For this review, use the dimensioned drawing (mm, ordinates from the lowest corner) and the shaded views. Coordinates: 2 decimals unless noted, no trailing zeros. Order: outer loops, then holes, each group sorted by start corner. A loop starts at its lowest first (then second) coordinate and runs counter-clockwise, first axis right, second up. Notation, with made-up numbers: (49, 7) -> (86, 7) arc R31 cw to (86, 34) -> close; hole circle Ø4 at (14.25, 42.25). An arc over 180 degrees is marked (long way). Return JSON: item names as keys, results as strings. Group by question number.
Item 1: For line 1 along Y through (x, z) = (44, 28); line 2 along Z through (x, y) = (10, 2.5); line 3 along X through (y, z) = (1.8, 44), list the stretches that pass through material, from the lowest coordinate up.
Item 2: Take a section at A-A (x = 25). Write out the cut boundary in (y, z).
Item 3: Take a section at C-C (z = 25). Write out the cut boundary in (x, y).
Item 4: Take a section at D-D (y = 7.75). Write out the cut boundary in (x, z).
Item 5: Draft analysis for pull direction X (two halves, no side actions). For the marked faces 1, 2 and 3, state which applies: +X half, -X half, draft (parallel to the pull), parting line (faces both ways), or undercut.
Item 6: Insertion check: pin 1 (4 mm diameter, centred on x = 6, z = 25, fed in from -Y); pin 2 (5 mm diameter, centred on x = 25, z = 6, fed in from +Y); pin 3 (1 mm diameter, centred on x = 40.5, y = 2, fed in from -Z); pin 4 (6 mm diameter, centred on x = 31.5, y = 3.5, fed in from -Z). Each pin has a flat end and moves straight along its axis. Give the tip position at first contact, or say it passes through.
Item 7: Take a section at B-B (z = 44). Write out the cut boundary in (x, y), then the cut area to 3 significant figures.
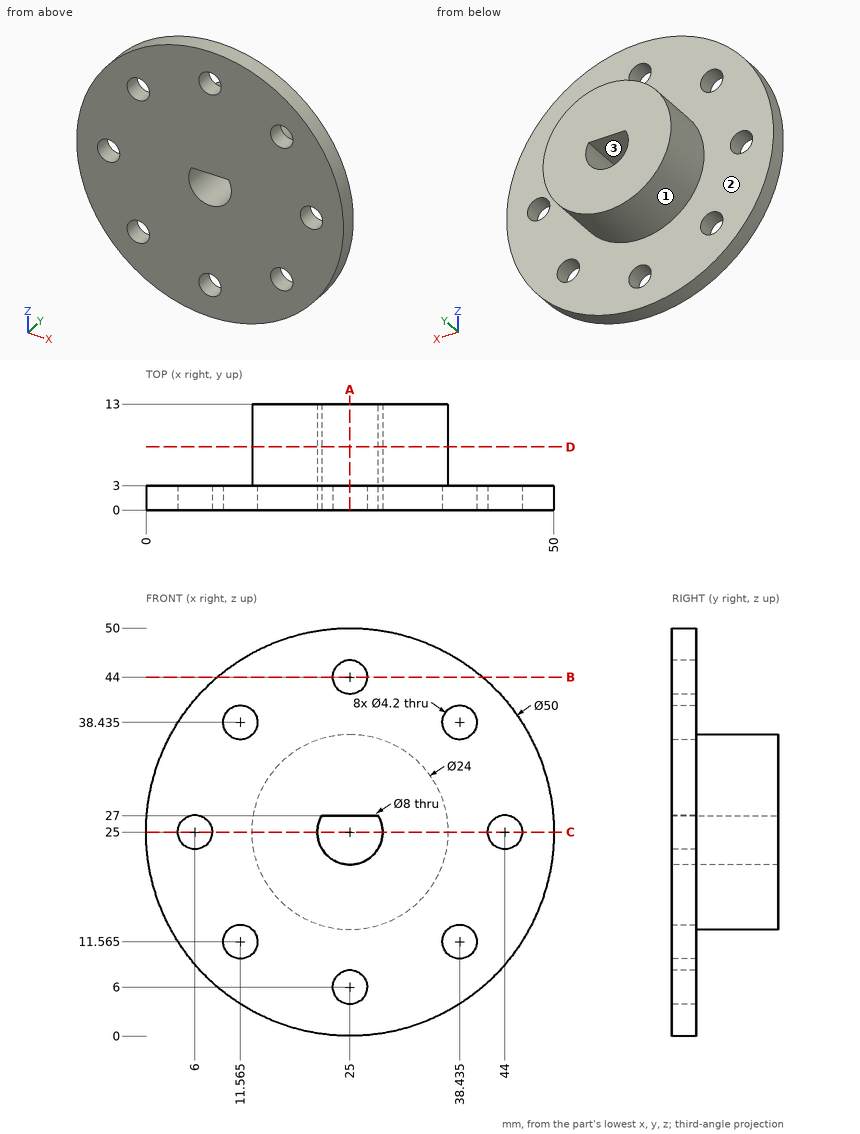
Findings below:
{
 "1": {"line 1": "y = 0 to 3", "line 2": "z = 5 to 10.16, 12.97 to 37.03, 39.84 to 45", "line 3": "x = 8.75 to 22.9, 27.1 to 41.25"},
 "2": {"outline": "(0, 0) -> (3, 0) -> (3, 3.9) -> (0, 3.9) -> close; (0, 8.1) -> (3, 8.1) -> (3, 13) -> (13, 13) -> (13, 21) -> (0, 21) -> close; (0, 27) -> (13, 27) -> (13, 37) -> (3, 37) -> (3, 41.9) -> (0, 41.9) -> close; (0, 46.1) -> (3, 46.1) -> (3, 50) -> (0, 50) -> close"},
 "3": {"outline": "(0, 0) -> (3.9, 0) -> (3.9, 3) -> (0, 3) -> close; (8.1, 0) -> (21, 0) -> (21, 13) -> (13, 13) -> (13, 3) -> (8.1, 3) -> close; (29, 0) -> (41.9, 0) -> (41.9, 3) -> (37, 3) -> (37, 13) -> (29, 13) -> close; (46.1, 0) -> (50, 0) -> (50, 3) -> (46.1, 3) -> close"},
 "4": {"outline": "circle Ø24 at (25, 25); hole (21.54, 27) arc R4 ccw (long way) to (28.46, 27) -> close"},
 "5": {"face 1": "parting line", "face 2": "draft", "face 3": "undercut"},
 "6": {"pin 1": "passes through", "pin 2": "stops at y = 3", "pin 3": "stops at z = 5", "pin 4": "stops at z = 0.25"},
 "7": {"outline": "(8.75, 0) -> (22.9, 0) -> (22.9, 3) -> (8.75, 3) -> close; (27.1, 0) -> (41.25, 0) -> (41.25, 3) -> (27.1, 3) -> close", "area": "84.9 mm2"}
}
